from build123d import *

# Parameters (mm, degrees)
SKETCH1_R               = 1.621
BASENUT_DEPTH           = 3.2
ENDCHAMFER_SIZE         = 0.379
ENDCHAMFER_SIZE2        = 0.218815752
ENDCHAMFER_PART_2_SIZE  = 0.379
ENDCHAMFER_PART_2_SIZE2 = 0.218815752


with BuildPart() as part:
    # Sketch1 → BaseNut (new body)
    with BuildSketch(Plane.XY):
        Polygon((4.041451884, 0), (2.020725942, 3.5), (-2.020725942, 3.5), (-4.041451884, 0), (-2.020725942, -3.5), (2.020725942, -3.5), align=None)
        Circle(SKETCH1_R, mode=Mode.SUBTRACT)
    extrude(amount=-BASENUT_DEPTH)

    # Sketch2 → Double-Chamfer (revolve, cut)
    with BuildSketch(Plane(origin=(0, 0, 0), x_dir=(1, 0, 0), z_dir=(0, 1, 0))):
        Polygon((-4.041451884, 3.2), (-3.125, 3.2), (-4.041451884, 2.670886258), align=None)
        Polygon((-4.041451884, 0.529113742), (-4.041451884, 0), (-3.125, 0), align=None)
    revolve(axis=Axis((0, 0, -3.375940562), (0, 0, 1)), mode=Mode.SUBTRACT)

    # EndChamfer
    endchamfer_edges = [part.edges().sort_by_distance(p)[0] for p in [
        (-1.621, 0, -3.2),
    ]]
    endchamfer_side = [part.faces().sort_by_distance(p)[0] for p in [
        (-1.621, 0, -1.6),
    ]]
    chamfer(endchamfer_edges, length=ENDCHAMFER_SIZE, length2=ENDCHAMFER_SIZE2, reference=endchamfer_side[0])

    # EndChamfer part 2
    endchamfer_part_2_edges = [part.edges().sort_by_distance(p)[0] for p in [
        (-1.621, 0, 0),
    ]]
    endchamfer_part_2_side = [part.faces().sort_by_distance(p)[0] for p in [
        (3.036611652, 0, 0),
    ]]
    chamfer(endchamfer_part_2_edges, length=ENDCHAMFER_PART_2_SIZE, length2=ENDCHAMFER_PART_2_SIZE2, reference=endchamfer_part_2_side[0])


solid = part.part
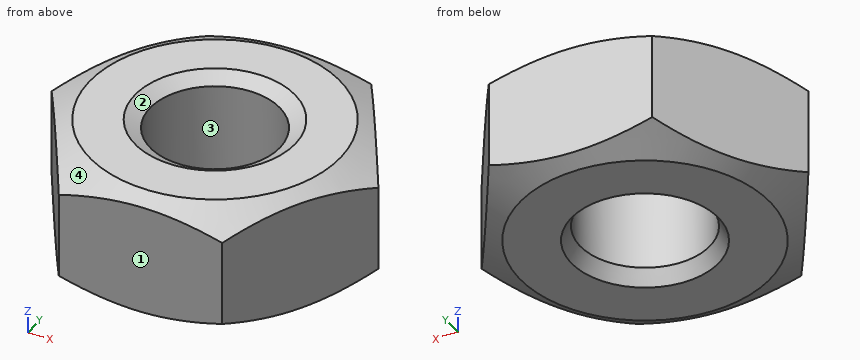
Model file for the job. Use its own axes, mm. Face numbers are marked on the shaded views. Give positions to 0.01 mm unless a question says otherwise; leave off trailing zeros. Loops run counter-clockwise (first coordinate to the right, second up) from the corner with the lowest first, then second, coordinate; pieces in that order, holes last.
Item 1: Drill centre lines: line 1 along Y through (x, z) = (0, -2); line 2 along X through (y, z) = (0.5, -2.45); line 3 along Y through (x, z) = (1.5, -2.95). Where is each one in solid material? Low to high.
Check values:
line 1: y = -3.5 to -1.62, 1.62 to 3.5
line 2: x = -3.75 to -1.54, 1.54 to 3.75
line 3: y = -3.23 to -0.79, 0.79 to 3.23
Item 2: Slice it at A-A (x = 0). Write the cut outline in (y, z) (1 decimal).
Check values:
outline: (-3.5, -3) - (-3.1, -3.2) - (-1.8, -3.2) - (-1.6, -2.8) - (-1.6, -0.2) - (-2, 0) - (-3.1, 0) - (-3.5, -0.2) - close; (1.6, -2.8) - (1.8, -3.2) - (3.1, -3.2) - (3.5, -3) - (3.5, -0.2) - (3.1, 0) - (2, 0) - (1.6, -0.2) - close
Item 3: Mould opens along X. For the marked faces 1, 2, 3 and 4 say: +X half, -X half, draft (parallel to the pull), parting line (faces both ways), or undercut.
Check values:
face 1: draft
face 2: undercut
face 3: undercut
face 4: parting line
Item 4: Drop flat-ended pins along their axis: P1, Ø1, axis at y = -1, z = -1, coming from the +X side; P2, Ø3.5, axis at x = 0, y = 0, coming from the +Z side. Give the stop position or say it passes through.
Check values:
P1: stops at x = 3.75
P2: stops at z = -0.14
Item 5: Slice it at B-B (z = -1.9). Write the cut outline in (x, y).
Check values:
outline: (-4.04, 0) - (-2.02, -3.5) - (2.02, -3.5) - (4.04, 0) - (2.02, 3.5) - (-2.02, 3.5) - close; hole circle Ø3.24 at (0, 0)
